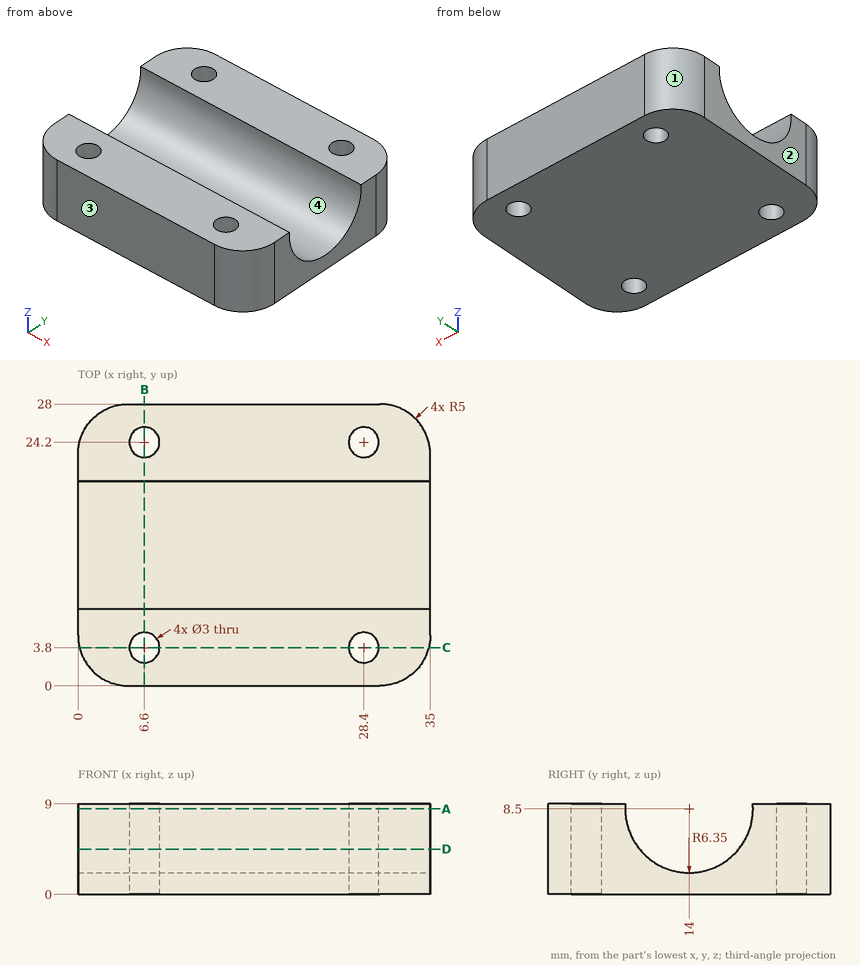
Here's the drawing with two shaded views (mm, measured from the low corner). I have some questions. Coordinates: 2 decimals unless noted, no trailing zeros. Order: outer loops, then holes, each group sorted by start corner. A loop starts at its lowest first (then second) coordinate and runs counter-clockwise, first axis right, second up. Notation, with made-up numbers: (76, 25.5) -> (101, 25.5) arc R10 cw to (101, 44.5) -> close; hole circle Ø10 at (18, 10). An arc over 180 degrees is marked (long way). One line per question, with ' | ' between items.
Q1. If I drill on L1, parallel to Y at x = 6.6, z = 2; L2, parallel to Y at x = 28.4, z = 6.75; L3, parallel to Y at x = 28.4, z = 7, over which ranges is the centre line in solid material (lowest first)?
Return value:
L1: 0 to 2.3, 5.3 to 22.7, 25.7 to 28 | L2: 0 to 2.3, 5.3 to 7.9, 20.1 to 22.7, 25.7 to 28 | L3: 0 to 2.3, 5.3 to 7.83, 20.17 to 22.7, 25.7 to 28
Q2. Imagine slicing it at B-B on x = 6.6. Please give me the cut outline in (y, z).
Return value:
outline: (0, 0) -> (2.3, 0) -> (2.3, 9) -> (0, 9) -> close; (5.3, 0) -> (22.7, 0) -> (22.7, 9) -> (20.33, 9) arc R6.35 cw (long way) to (7.67, 9) -> (5.3, 9) -> close; (25.7, 0) -> (28, 0) -> (28, 9) -> (25.7, 9) -> close
Q3. Imagine slicing it at A-A on z = 8.5. Please give me the cut outline in (x, y).
Return value:
outline: (0, 5) arc R5 ccw to (5, 0) -> (30, 0) arc R5 ccw to (35, 5) -> (35, 7.65) -> (0, 7.65) -> close; (0, 20.35) -> (35, 20.35) -> (35, 23) arc R5 ccw to (30, 28) -> (5, 28) arc R5 ccw to (0, 23) -> close; hole circle Ø3 at (6.6, 3.8); hole circle Ø3 at (6.6, 24.2); hole circle Ø3 at (28.4, 3.8); hole circle Ø3 at (28.4, 24.2)
Q4. Thinking about a two-plate mould opening in Y: for the marked faces 1, 2, 3 and 4, which applies, pulls with the +Y half, pulls with the -Y half, needs draft (parallel to the pull), parting line crosses it, or undercut?
Return value:
face 1: pulls with the +Y half | face 2: needs draft | face 3: pulls with the -Y half | face 4: undercut
Q5. Imagine slicing it at D-D on z = 4.5. Please give me the cut outline in (x, y).
Return value:
outline: (0, 5) arc R5 ccw to (5, 0) -> (30, 0) arc R5 ccw to (35, 5) -> (35, 9.07) -> (0, 9.07) -> close; (0, 18.93) -> (35, 18.93) -> (35, 23) arc R5 ccw to (30, 28) -> (5, 28) arc R5 ccw to (0, 23) -> close; hole circle Ø3 at (6.6, 3.8); hole circle Ø3 at (6.6, 24.2); hole circle Ø3 at (28.4, 3.8); hole circle Ø3 at (28.4, 24.2)
Q6. I'm going to push a flat-ended pin straight in: P1, Ø2, axis at x = 10.5, y = 12.5, coming from the -Z side. Where does the tip first touch, or does it pass through?
Return value:
P1: z = 0
Q7. Imagine slicing it at C-C on y = 3.8. Please give me the cut outline in (x, z).
Return value:
outline: (0.15, 0) -> (5.1, 0) -> (5.1, 9) -> (0.15, 9) -> close; (8.1, 0) -> (26.9, 0) -> (26.9, 9) -> (8.1, 9) -> close; (29.9, 0) -> (34.85, 0) -> (34.85, 9) -> (29.9, 9) -> close
